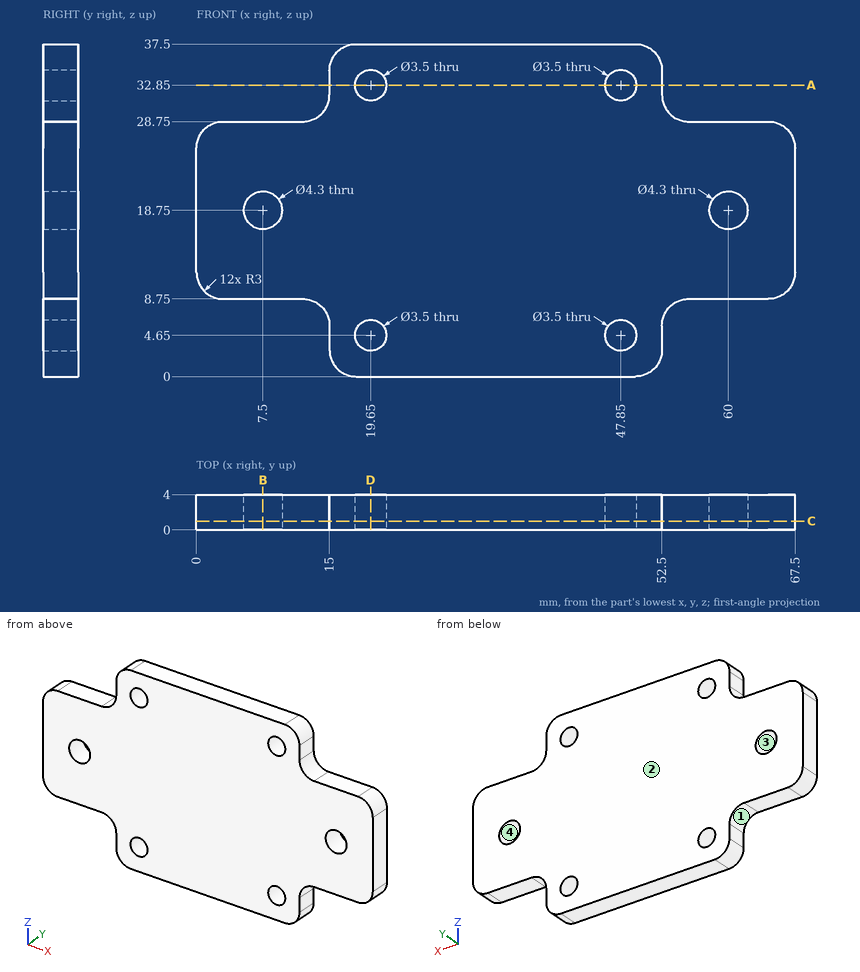
Here's the drawing with two shaded views (mm, measured from the low corner). I have some questions. Coordinates: 2 decimals unless noted, no trailing zeros. Order: outer loops, then holes, each group sorted by start corner. A loop starts at its lowest first (then second) coordinate and runs counter-clockwise, first axis right, second up. Notation, with made-up numbers: (26, -37.75) -> (41, -37.75) arc R35 ccw to (41, -5.75) -> close; hole circle Ø9 at (57, 88.5). An arc over 180 degrees is marked (long way). One line per question, with ' | ' between items.
Q1. Imagine slicing it at D-D on x = 19.65. Please give me the cut outline in (y, z).
Return value:
outline: (0, 0) -> (4, 0) -> (4, 2.9) -> (0, 2.9) -> close; (0, 6.4) -> (4, 6.4) -> (4, 31.1) -> (0, 31.1) -> close; (0, 34.6) -> (4, 34.6) -> (4, 37.5) -> (0, 37.5) -> close
Q2. I'm going to push flat-ended pins straight in: P1, Ø2, axis at y = 2, z = 3.5, coming from the -X side; P2, Ø5.5, axis at x = 19.65, z = 32.85, coming from the -Y side; P3, Ø2, axis at x = 6, y = 1, coming from the +Z side; P4, Ø0.8, axis at y = 1.5, z = 33, coming from the +X side. Where does each tip first touch, or does it pass through?
Return value:
P1: x = 15 | P2: y = 0 | P3: z = 28.75 | P4: x = 52.5
Q3. Thinking about a two-plate mould opening in Z: for the marked faces 1, 2, 3 and 4, which applies, pulls with the +Z half, pulls with the -Z half, needs draft (parallel to the pull), parting line crosses it, or undercut?
Return value:
face 1: pulls with the -Z half | face 2: needs draft | face 3: undercut | face 4: undercut
Q4. Imagine slicing it at C-C on y = 1. State how many separate pieces and enclosed holes the cut face has, and give its area (3 significant figures).
Return value:
separate pieces: 1 | enclosed holes: 6 | area: 1,930 mm²
Q5. Imagine slicing it at A-A on z = 32.85. Please give me the cut outline in (x, y).
Return value:
outline: (15, 0) -> (17.9, 0) -> (17.9, 4) -> (15, 4) -> close; (21.4, 0) -> (46.1, 0) -> (46.1, 4) -> (21.4, 4) -> close; (49.6, 0) -> (52.5, 0) -> (52.5, 4) -> (49.6, 4) -> close
Q6. Imagine slicing it at B-B on x = 7.5. Please give me the cut outline in (y, z), and give its area (3 significant figures).
Return value:
outline: (0, 8.75) -> (4, 8.75) -> (4, 16.6) -> (0, 16.6) -> close; (0, 20.9) -> (4, 20.9) -> (4, 28.75) -> (0, 28.75) -> close | area: 62.8 mm²
Q7. If I drill on L1, parallel to X at y = 1.6, z = 4.65; L2, parallel to Z at x = 47.85, y = 0.95; L3, parallel to X at y = 3.65, z = 19, over which ranges is the centre line in solid material (lowest first)?
Return value:
L1: 15 to 17.9, 21.4 to 46.1, 49.6 to 52.5 | L2: 0 to 2.9, 6.4 to 31.1, 34.6 to 37.5 | L3: 0 to 5.36, 9.64 to 57.86, 62.14 to 67.5
